```python
from build123d import *

# Parameters (mm, degrees)
F0_W      = 15.875
F0_H      = 4.953
F1_DEPTH  = 50.8
F3_DEPTH  = 50.8
F4_W      = 5.588
F4_H      = 3.175
F5_DEPTH  = 50.8
F6_W      = 5.588
F6_H      = 12.7
F7_DEPTH  = 3.175
F8_W      = 1.524
F8_H      = 1.27
F9_DEPTH  = 50.801
F11_DEPTH = 5.588
F12_W     = 4.3942
F12_H     = 5.3848
F13_DEPTH = 25.4
F14_SIZE  = 1.27
F15_SIZE  = 0.635


with BuildPart() as f1:
    # F0 (on Top) → F1 (new body)
    with BuildSketch(Plane.XY):
        with Locations((13.4436743471, 8.5170986131)):
            Rectangle(F0_W, F0_H)
    extrude(amount=F1_DEPTH)

    # F2 (on face) → F3 (join)
    with BuildSketch(Plane.XY.offset(50.8)):
        Polygon((3.9186743471, 12.5810986131), (5.5061743471, 10.9935986131), (21.3811743471, 10.9935986131), (22.9686743471, 12.5810986131), (22.9686743471, 13.8002986131), (21.3811743471, 15.3877986131), (5.5061743471, 15.3877986131), (3.9186743471, 13.8002986131), align=None)
    extrude(amount=-F3_DEPTH)

    # F4 (on face) → F5 (join, through all)
    with BuildSketch(Plane.XY.offset(50.8)):
        with Locations((13.4436743471, 4.4530986131)):
            Rectangle(F4_W, F4_H)
    extrude(amount=-F5_DEPTH)

    # F6 (on face) → F7 (cut, through all)
    with BuildSketch(Plane.XZ.offset(-2.8655986131)):
        with Locations((13.4436743471, 25.4)):
            Rectangle(F6_W, F6_H)
    extrude(amount=-F7_DEPTH, mode=Mode.SUBTRACT)

    # F8 (on face) → F9 (cut, through all)
    with BuildSketch(Plane(origin=(0, 0, 0), x_dir=(1, 0, 0), z_dir=(0, 0, -1))):
        with Locations((15.4756743471, -5.4055986131)):
            Rectangle(F8_W, F8_H)
        with Locations((11.4116743471, -5.4055986131)):
            Rectangle(F8_W, F8_H)
    extrude(amount=-F9_DEPTH, mode=Mode.SUBTRACT)

    # F10 (on face) → F11 (cut, through all)
    with BuildSketch(Plane.YZ.offset(16.2376743471)):
        Polygon((6.0405986131, 0), (2.8655986131, 3.4018158913), (2.8655986131, 0), align=None)
        Polygon((6.0405986131, 31.75), (2.8655986131, 34.2048890889), (2.8655986131, 31.75), align=None)
    extrude(amount=-F11_DEPTH, mode=Mode.SUBTRACT)

    # F12 (on face) → F13 (cut, symmetric)
    with BuildSketch(Plane.YZ.offset(21.3811743471)):
        with Locations((13.1906986131, 42.7228)):
            Rectangle(F12_W, F12_H)
        with Locations((13.1906986131, 31.9532)):
            Rectangle(F12_W, F12_H)
        with Locations((13.1906986131, 21.1836)):
            Rectangle(F12_W, F12_H)
        with Locations((13.1906986131, 10.414)):
            Rectangle(F12_W, F12_H)
    extrude(amount=F13_DEPTH, both=True, mode=Mode.SUBTRACT)

    # F14
    f14_edges = [f1.edges().sort_by_distance(p)[0] for p in [
        (13.443674, 10.993599, 7.7216),
        (13.443674, 10.993599, 13.1064),
        (13.443674, 10.993599, 18.4912),
        (13.443674, 10.993599, 23.876),
        (13.443674, 10.993599, 29.2608),
        (13.443674, 10.993599, 34.6456),
        (13.443674, 10.993599, 40.0304),
        (13.443674, 10.993599, 45.4152),
    ]]
    chamfer(f14_edges, length=F14_SIZE)

    # F15
    f15_edges = [f1.edges().sort_by_distance(p)[0] for p in [
        (13.443674, 15.387799, 34.6456),
        (13.443674, 15.387799, 23.876),
        (13.443674, 15.387799, 13.1064),
        (13.443674, 15.387799, 45.4152),
        (22.174924, 14.594049, 45.4152),
        (22.174924, 14.594049, 34.6456),
        (22.174924, 14.594049, 23.876),
        (22.174924, 14.594049, 13.1064),
        (4.712424, 14.594049, 13.1064),
        (4.712424, 14.594049, 23.876),
        (4.712424, 14.594049, 34.6456),
        (4.712424, 14.594049, 45.4152),
    ]]
    chamfer(f15_edges, length=F15_SIZE)


solid = f1.part
```
Source: CAD feature listing. Evaluate the final solid. Frame: model axes, mm. A direction names the side the tool comes from. Give positions to 0.01 mm unless a question says otherwise; leave off trailing zeros. Loops run counter-clockwise (first coordinate to the right, second up) from the corner with the lowest first, then second, coordinate; pieces in that order, holes last. Notation, with made-up numbers: (18, 33.5) - (72, 33.5) arc R17 ccw to (72, 42.5) - close; hole circle Ø5 at (34.5, 9.5). An arc over 180 degrees is marked (long way). Use CSV: the item, a comma, the result in double quotes. Start each with the question number.
1. Section A-A (z = 14.5). Output: boundary loops of the cut face in (x, y), then the cut area to 3 significant figures.
2. Ray query, L1, parallel to Z at x = 21.75, y = 13; L2, parallel to Z at x = 20, y = 11.75; L3, parallel to Y at x = 15, z = 48. Return the intervals inside material, ascending.
3. Reachability of faces 1 (the flat face through (4.7, 14.13, 45.73)), 2 (the flat face through (10.65, 4, 42)), 3 (the flat face through (13.315, 11.637, 29.887)), 4 (the flat face through (16.238, 4, 42)) from +Z, -Z, +X, -X, +Y, -Y: full face, straight path, thin tool, end or side. Return the list, or none.
4. Section D-D (x = 15.5). Count the separate pieces of the cut face and the enclosed holes in it, then the cut area to 3 significant figures.
5. Pin query (flat end, axial travel): pin 1 (0.5 mm diameter, centred on x = 11.5, z = 9, fed in from +Y); pin 2 (2 mm diameter, centred on y = 12.5, z = 42.5, fed in from +X); pin 3 (0.6 mm diameter, centred on y = 3.5, z = 13.5, fed in from +X); pin 4 (2 mm diameter, centred on x = 19, z = 41.5, fed in from -Y). Return the tip coordinate at first contact, or that it passes through.
6. Section C-C (y = 6.5). Output: boundary loops of the cut face in (x, z), then the cut area to 3 significant figures.
7. Draft query along Y for faces 5 (the flat face through (12.174, 5, 41)), 6 (the flat face through (4.7, 11.8, 48.3)), 7 (the flat face through (4.724, 14.605, 48.458)), 8 (the flat face through (11, 4.771, 42)). Return one class per face: +Y half, -Y half, draft (parallel to the pull), parting line (faces both ways), or undercut.
Response:
1,outline,"(3.92, 12.58) - (5.51, 10.99) - (5.51, 6.04) - (12.17, 6.04) - (12.17, 4.77) - (10.65, 4.77) - (10.65, 2.87) - (16.24, 2.87) - (16.24, 4.77) - (14.71, 4.77) - (14.71, 6.04) - (21.38, 6.04) - (21.38, 10.99) - (22.97, 12.58) - (22.97, 13.8) - (21.38, 15.39) - (5.51, 15.39) - (3.92, 13.8) - close"
1,area,"171 mm²"
2,L1,"0 to 7.72, 13.11 to 18.49, 23.88 to 29.26, 34.65 to 40.03, 45.42 to 50.8"
2,L2,"0 to 8.24, 12.59 to 19, 23.36 to 29.77, 34.13 to 40.54, 44.9 to 50.8"
2,L3,"2.87 to 4.77, 6.04 to 15.39"
3,face 1,"-X, +Y"
3,face 2,"+Z, -Z, -X, -Y"
3,face 3,"+X, -X, +Y"
3,face 4,"+Z, -Z, +X, -Y"
4,separate pieces,"3"
4,enclosed holes,"0"
4,area,"451 mm²"
5,pin 1,"y = 11.24"
5,pin 2,"through"
5,pin 3,"x = 16.24"
5,pin 4,"y = 6.04"
6,outline,"(5.51, 0) - (21.38, 0) - (21.38, 50.8) - (5.51, 50.8) - close"
6,area,"806 mm²"
7,face 5,"undercut"
7,face 6,"-Y half"
7,face 7,"+Y half"
7,face 8,"undercut"
